from build123d import *

# Parameters (mm, degrees)
SKETCH1_W           = 180
SKETCH1_H           = 20
BOSS_EXTRUDE1_DEPTH = 10
CUT_EXTRUDE2_DEPTH  = 4


with BuildPart() as part:
    # Sketch1 → Boss-Extrude1 (new body)
    with BuildSketch(Plane(origin=(0, 0, 0), x_dir=(1, 0, 0), z_dir=(0, 1, 0))):
        Rectangle(SKETCH1_W, SKETCH1_H)
    extrude(amount=BOSS_EXTRUDE1_DEPTH)

    # Sketch2 → Cut-Extrude2 (cut)
    with BuildSketch(Plane(origin=(0, 10, 0), x_dir=(1, 0, 0), z_dir=(0, 1, 0))):
        Polygon((84.5, -2), (84.5, -7.781340665), (84.5, -10), (82.5, -10), (82.5, -8), (75.5, -8), (75.5, -2), align=None)
        Polygon((44.5, -2), (44.5, -7.781340665), (44.5, -10), (42.5, -10), (42.5, -8), (35.5, -8), (35.5, -2), align=None)
        Polygon((4.5, -2), (4.5, -7.781340665), (4.5, -10), (2.5, -10), (2.5, -8), (-4.5, -8), (-4.5, -2), align=None)
        Polygon((-35.5, -2), (-35.5, -7.781340665), (-35.5, -10), (-37.5, -10), (-37.5, -8), (-44.5, -8), (-44.5, -2), align=None)
        Polygon((-75.5, -2), (-75.5, -7.781340665), (-75.5, -10), (-77.5, -10), (-77.5, -8), (-84.5, -8), (-84.5, -2), align=None)
    extrude(amount=-CUT_EXTRUDE2_DEPTH, mode=Mode.SUBTRACT)


solid = part.part
The model under review builds one solid part; all positions refer to its coordinate system, in mm. A direction names the side the tool comes from. Round coordinates to 2 decimals unless told otherwise and drop trailing zeros. Write each loop counter-clockwise with the first axis right and the second up, starting at its lowest first coordinate (ties: lowest second). Pieces come first, ordered by that corner, then holes. Notation, with made-up numbers: M 48,39 L 84,39 A22 cw 84,75 Z; hole C 83.5,52 d1. An arc over 180 degrees is marked long. Answer as CSV lines item,"result". Start each with the question number.
Q1. Wall thickness on line 1 along X through (y, z) = (7, 7.75); line 2 along Z through (x, y) = (4, 8.5); line 3 along Y through (x, z) = (1, 5.25): over which ranges is each line inside the solid? List them lowest first.
Q2. Tool access review of faces 1 (the face through (-1, 5, -10)), 2 (the face through (35.5, 8, 5)), 3 (the face through (4.5, 8, 6)): name each direction out of +Z, -Z, +X, -X, +Y, -Y from which nothing blocks a thin tool from reaching the whole face with its end or side.
Q3. Clearance check with flat-ended pins moving along their axes: P1, Ø6.5, axis at x = -79.5, z = 4.5, coming from the +Y side; P2, Ø4, axis at x = 2, z = 5.5, coming from the +Y side. State where each tip first meets the part, or that it passes through.
Q4. The part is to be moulded in two halves that separate along X. For faces 4 (the face through (-1, 10, 0)), 5 (the face through (-75.5, 8, 6)), say which applies: +X half, -X half, draft (parallel to the pull), parting line (faces both ways), or undercut.
Q5. Consider section A-A, the plane x = -42. Give the boundary of the cut face in (y, z), then the cut area to 3 significant figures.
Result set:
1,line 1,"x = -90 to -84.5, -75.5 to -44.5, -35.5 to -4.5, 4.5 to 35.5, 44.5 to 75.5, 84.5 to 90"
1,line 2,"z = -10 to 2"
1,line 3,"y = 0 to 6"
2,face 1,"-Z, +X, -X, +Y, -Y"
2,face 2,"+Y"
2,face 3,"+Z, +Y"
3,P1,"stops at y = 10"
3,P2,"stops at y = 6"
4,face 4,"draft"
4,face 5,"undercut"
5,outline,"M 0,-10 L 10,-10 L 10,2 L 6,2 L 6,8 L 10,8 L 10,10 L 0,10 Z"
5,area,"176 mm²"
